Here's how the part is built. I have some questions about the finished solid (model axes, mm). Face numbers are marked on the shaded views. Give positions to 0.01 mm unless a question says otherwise; leave off trailing zeros. Write each loop counter-clockwise with the first axis right and the second up, starting at its lowest first coordinate (ties: lowest second). Pieces come first, ordered by that corner, then holes. Notation, with made-up numbers: M 66,52 L 72,52 A24 cw 72,75 Z; hole C 75,89 d4. An arc over 180 degrees is marked long. Use one line per item in the form item = value. Start each with the question number.
from build123d import *

# Parameters (mm, degrees)
SKETCH4_W                    = 133.35
SKETCH4_H                    = 249.936
BOSS_EXTRUDE2_DEPTH          = 1.5875
EDGE_FLANGE1_STRIP_W         = 14.1732
EDGE_FLANGE1_STRIP_H         = 3.175
EDGE_FLANGE1_STRIP_CUT_DEPTH = 249.936
EDGE_FLANGE1_DEPTH           = 249.936
EDGE_FLANGE2_STRIP_W         = 14.1732
EDGE_FLANGE2_STRIP_H         = 3.175
EDGE_FLANGE2_STRIP_CUT_DEPTH = 249.936
EDGE_FLANGE2_DEPTH           = 249.936
SKETCH18_R                   = 3.2639
CUT_EXTRUDE1_DEPTH           = 213.759580995
SKETCH20_R                   = 12.7
CUT_EXTRUDE2_DEPTH           = 213.759580995


# Sheet-metal steps are written as plain solids
with BuildPart() as part:
    # Sketch4 → Boss-Extrude2 (new, symmetric)
    with BuildSketch(Plane(origin=(0, 0, 0), x_dir=(1, 0, 0), z_dir=(0, 1, 0))):
        Rectangle(SKETCH4_W, SKETCH4_H)
    extrude(amount=BOSS_EXTRUDE2_DEPTH, both=True)

    # Edge-Flange1 strip (across the edge) → Edge-Flange1 strip cut (cut)
    with BuildSketch(Plane(origin=(-66.675, 1.5875, -124.968), x_dir=(1, 0, 0), z_dir=(0, 0, 1))):
        with Locations((-3.175, -1.5875)):
            Rectangle(EDGE_FLANGE1_STRIP_W, EDGE_FLANGE1_STRIP_H)
    extrude(amount=EDGE_FLANGE1_STRIP_CUT_DEPTH, mode=Mode.SUBTRACT)

    # Edge-Flange1 section (across the edge) → Edge-Flange1 (add)
    with BuildSketch(Plane(origin=(-66.675, 1.5875, -124.968), x_dir=(1, 0, 0), z_dir=(0, 0, 1))):
        with BuildLine():
            Line((0, 0.7366), (0, 111.125))
            Line((0, 111.125), (3.175, 111.125))
            Line((3.175, 111.125), (3.175, 0.7366))
            ThreePointArc((3.175, 0.7366), (3.390745145, 0.215745145), (3.9116, 0))
            Line((3.9116, 0), (3.9116, -3.175))
            ThreePointArc((3.9116, -3.175), (1.145681115, -2.029318885), (0, 0.7366))
        make_face()
    extrude(amount=EDGE_FLANGE1_DEPTH)

    # Edge-Flange2 strip (across the edge) → Edge-Flange2 strip cut (cut)
    with BuildSketch(Plane(origin=(66.675, 1.5875, 124.968), x_dir=(-1, 0, 0), z_dir=(0, 0, -1))):
        with Locations((-3.175, -1.5875)):
            Rectangle(EDGE_FLANGE2_STRIP_W, EDGE_FLANGE2_STRIP_H)
    extrude(amount=EDGE_FLANGE2_STRIP_CUT_DEPTH, mode=Mode.SUBTRACT)

    # Edge-Flange2 section (across the edge) → Edge-Flange2 (add)
    with BuildSketch(Plane(origin=(66.675, 1.5875, 124.968), x_dir=(-1, 0, 0), z_dir=(0, 0, -1))):
        with BuildLine():
            Line((0, 0.7366), (0, 9.525))
            Line((0, 9.525), (3.175, 9.525))
            Line((3.175, 9.525), (3.175, 0.7366))
            ThreePointArc((3.175, 0.7366), (3.390745145, 0.215745145), (3.9116, 0))
            Line((3.9116, 0), (3.9116, -3.175))
            ThreePointArc((3.9116, -3.175), (1.145681115, -2.029318885), (0, 0.7366))
        make_face()
    extrude(amount=EDGE_FLANGE2_DEPTH)

    # Sketch18 → Cut-Extrude1 (cut, through all)
    with BuildSketch(Plane(origin=(-63.5, 0, 0), x_dir=(0, 0, -1), z_dir=(1, 0, 0))):
        with Locations(Location((-50.8, 100.0125, 0), (0, 0, 90))):
            Circle(SKETCH18_R)
        with Locations(Location((50.8, 100.0125, 0), (0, 0, 270))):
            Circle(SKETCH18_R)
        with Locations(Location((0, 100.0125, 0), (0, 0, 90))):
            Circle(SKETCH18_R)
    extrude(amount=-CUT_EXTRUDE1_DEPTH, mode=Mode.SUBTRACT)

    # Sketch20 → Cut-Extrude2 (cut, through all)
    with BuildSketch(Plane(origin=(-63.5, 0, 0), x_dir=(0, 0, -1), z_dir=(1, 0, 0))):
        with Locations((-74, 122.2375)):
            Circle(SKETCH20_R)
        with Locations((74, 122.2375)):
            Circle(SKETCH20_R)
    extrude(amount=-CUT_EXTRUDE2_DEPTH, mode=Mode.SUBTRACT)


solid = part.part
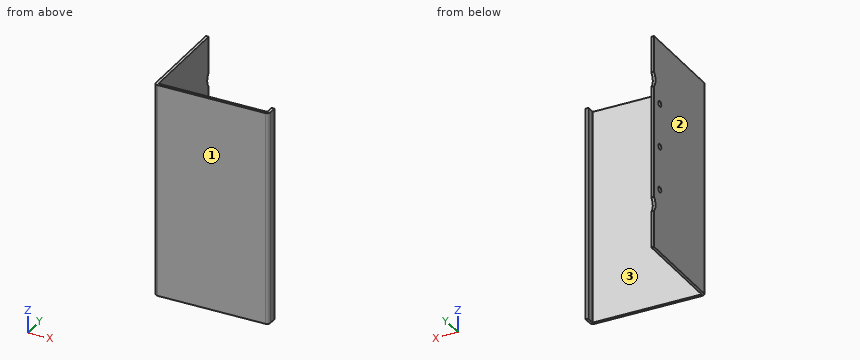
1) Please list where these lines run through material, in increasing order: line 1 (X direction, y = 9.5, z = 55.5) (3 decimals); line 2 (X direction, y = 84.5, z = 27) (3 decimals); line 3 (Y direction, x = -41, z = 76).
2) Will these pins go through, and if not, where does the flat tip stop? P1, Ø12, axis at y = 67, z = -59, coming from the +X side; P2, Ø7.5, axis at y = 100.01, z = 50.8, coming from the -X side (3 decimals); P3, Ø1.6, axis at x = 65, z = 44, coming from the +Y side; P4, Ø2, axis at x = 38.5, z = -64.5, coming from the +Y side.
3) Suppose I cut it at C-C, the plane x = -27.5. List the corners of the cut face in (y, z) for me.
4) Thinking about a two-plate mould opening in X: for the marked faces 1, 2 and 3, which applies, released by +X, released by -X, zero draft, split by the parting line, or undercut?
5) Suppose I cut it at A-A, the plane z = 0. List the corners of the cut face in (x, y) for me (1 decimal), and give its area (3 significant figures).
6) Suppose I cut it at B-B, the plane z = 74. List the corners of the cut face in (x, y) for me (1 decimal), and give its area (3 significant figures).
7) Suppose I cut it at D-D, the plane y = 65.5. List the corners of the cut face in (x, z) for me (3 decimals).
Checks:
q1.line_1 = -66.675 to -63.5, 63.5 to 66.675
q1.line_2 = -66.675 to -63.5
q1.line_3 = -1.59 to 1.59
q2.P1 = -63.5
q2.P2 = -66.675
q2.P3 = 11.11
q2.P4 = 1.59
q3.outline = M -1.59,-124.97 L 1.59,-124.97 L 1.59,124.97 L -1.59,124.97 Z
q4.face_1 = zero draft
q4.face_2 = released by -X
q4.face_3 = undercut
q5.outline = M -66.7,2.3 A3.9 ccw -62.8,-1.6 L 62.8,-1.6 A3.9 ccw 66.7,2.3 L 66.7,11.1 L 63.5,11.1 L 63.5,2.3 A0.7 cw 62.8,1.6 L -62.8,1.6 A0.7 cw -63.5,2.3 L -63.5,96.7 L -66.7,96.7 Z; M -66.7,103.3 L -63.5,103.3 L -63.5,112.7 L -66.7,112.7 Z
q5.area = 779 mm^2
q6.outline = M -66.7,2.3 A3.9 ccw -62.8,-1.6 L 62.8,-1.6 A3.9 ccw 66.7,2.3 L 66.7,11.1 L 63.5,11.1 L 63.5,2.3 A0.7 cw 62.8,1.6 L -62.8,1.6 A0.7 cw -63.5,2.3 L -63.5,109.5 L -66.7,109.5 Z
q6.area = 790 mm^2
q7.outline = M -66.675,-124.968 L -63.5,-124.968 L -63.5,124.968 L -66.675,124.968 Z
